For this review, take the finished solid that the model builds, in its own axes (mm). Face numbers are marked on the shaded views. A direction names the side the tool comes from. Coordinates: 2 decimals unless noted, no trailing zeros. Loops run counter-clockwise (first coordinate to the right, second up) from the corner with the lowest first, then second, coordinate; pieces in that order, holes last. Notation, with made-up numbers: (-16, 40.25) -> (39, 40.25) arc R21 ccw to (39, 77.25) -> close; hole circle Ø5 at (50.25, -38.75). An arc over 180 degrees is marked (long way). Answer in a Markdown table with one row per item.
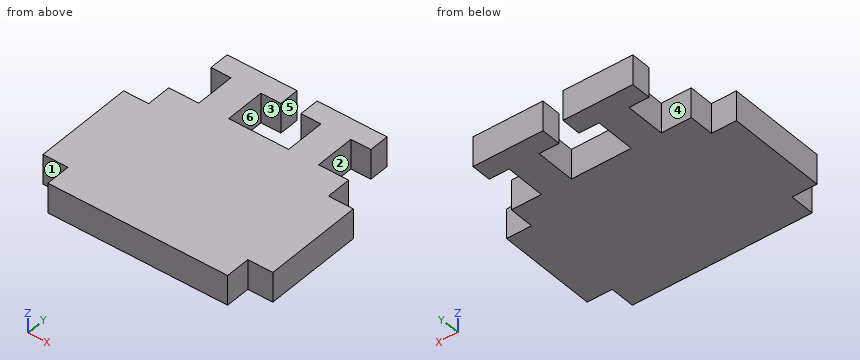
Autodesk Inventor part; units mm, degrees
ref_plane "YZ Plane" through (0, 0, 0) normal (1, 0, 0) x (0, 1, 0)
ref_plane "XZ Plane" through (0, 0, 0) normal (0, 1, 0) x (-1, 0, 0)
ref_plane "XY Plane" through (0, 0, 0) normal (0, 0, 1) x (1, 0, 0)
sketch "Sketch1" plane through (0, 0, 0) normal (0, 0, 1) x (1, 0, 0)
  line L0 (0, 0) -> (18, 0)
  line L1 (18, 0) -> (18, 15)
  line L2 (18, 15) -> (0, 15)
  line L3 (0, 15) -> (0, 0)
  line L4 (20.5, 12.5) -> (18, 12.5)
  line L5 (18, 12.5) -> (18, 2.5)
  line L6 (18, 2.5) -> (20.5, 2.5)
  line L7 (20.5, 2.5) -> (20.5, 12.5)
  line L8 (20.5, 12.5) -> (18, 2.5) construction
  line L9 (18, 12.5) -> (20.5, 2.5) construction
  line L10 (-2.5, 12.5) -> (0, 12.5)
  line L11 (0, 12.5) -> (0, 2.5)
  line L12 (0, 2.5) -> (-2.5, 2.5)
  line L13 (-2.5, 2.5) -> (-2.5, 12.5)
  line L14 (-2.5, 12.5) -> (0, 2.5) construction
  line L15 (0, 12.5) -> (-2.5, 2.5) construction
  line L16 (3, 15) -> (3, 19)
  line L17 (3, 19) -> (1, 19)
  line L18 (1, 19) -> (1, 21)
  line L19 (1, 21) -> (8, 21)
  line L20 (8, 21) -> (8, 19)
  line L21 (8, 19) -> (6, 19)
  line L22 (6, 19) -> (6, 15)
  line L23 (12, 15) -> (12, 19)
  line L24 (12, 19) -> (10, 19)
  line L25 (10, 19) -> (10, 21)
  line L26 (10, 21) -> (17, 21)
  line L27 (17, 21) -> (17, 19)
  line L28 (17, 19) -> (15, 19)
  line L29 (15, 19) -> (19.0944, 19)
  line L30 (15, 19) -> (15, 15)
  point P0 (19.25, 7.5)
  point P1 (-1.25, 7.5)
  point P2 (18, 7.5)
  point P3 (0, 7.5)
  point P4 (0, 12.5)
  dimension "d0" = 18
  dimension "d1" = 15
  dimension "d2" = 2.5
  dimension "d3" = 2.5
  dimension "d4" = 10
  dimension "d5" = 4
  dimension "d6" = 2
  dimension "d7" = 2
  dimension "d8" = 7
  dimension "d9" = 2
  dimension "d10" = 2
  dimension "d11" = 3
  dimension "d21" = 4
  dimension "d22" = 2
  dimension "d23" = 2
  dimension "d24" = 7
  dimension "d25" = 2
  dimension "d26" = 2
  dimension "d27" = 3
extrude "Extrusion1" add sketch "Sketch1" along normal blind 3
properties part number "Spring_holder2"
Item 1: Take a section at A-A, the plane y = 17.75. State the section outline as (x, z) points.
Worked answers:
| item | result |
|---|---|
| outline | (3, 0) -> (6, 0) -> (6, 3) -> (3, 3) -> close; (12, 0) -> (15, 0) -> (15, 3) -> (12, 3) -> close |
Item 2: The part is to be moulded in two halves that separate along X. For the marked faces 1, 2 and 3, say which applies: +X half, -X half, draft (parallel to the pull), parting line (faces both ways), or undercut.
Worked answers:
| item | result |
|---|---|
| face 1 | draft |
| face 2 | +X half |
| face 3 | undercut |
Item 3: Take a section at B-B, the plane x = 7.25. State the section outline as (y, z) points.
Worked answers:
| item | result |
|---|---|
| outline | (0, 0) -> (15, 0) -> (15, 3) -> (0, 3) -> close; (19, 0) -> (21, 0) -> (21, 3) -> (19, 3) -> close |
Item 4: Take a section at D-D, the plane y = 13.25. State the section outline as (x, z) points, and give its area (3 significant figures).
Worked answers:
| item | result |
|---|---|
| outline | (0, 0) -> (18, 0) -> (18, 3) -> (0, 3) -> close |
| area | 54.0 mm² |
Item 5: Insertion check: pin 1 (1.5 mm diameter, centred on y = 16.5, z = 1, fed in from -X); pin 2 (1.5 mm diameter, centred on y = 18, z = 1, fed in from +X); pin 3 (1 mm diameter, centred on y = 20, z = 1.5, fed in from -X); pin 4 (1 mm diameter, centred on x = 11, z = 1.5, fed in from -Y). Each pin has a flat end and moves straight along its axis. Give the tip position at first contact, or say it passes through.
Worked answers:
| item | result |
|---|---|
| pin 1 | x = 3 |
| pin 2 | x = 15 |
| pin 3 | x = 1 |
| pin 4 | y = 0 |
Item 6: For the marked faces 4, 5 and 6, list the 3-axis set-ups (+Z, -Z, +X, -X, +Y, -Y) from which the entire face can be reached by the end or side of a thin tool; tool diameter is ignored.
Worked answers:
| item | result |
|---|---|
| face 4 | +Z, -Z, -X |
| face 5 | +Z, -Z, +Y |
| face 6 | +Z, -Z |
Item 7: Take a section at C-C, the plane z = 1.55. State the section outline as (x, y) points.
Worked answers:
| item | result |
|---|---|
| outline | (-2.5, 2.5) -> (0, 2.5) -> (0, 0) -> (18, 0) -> (18, 2.5) -> (20.5, 2.5) -> (20.5, 12.5) -> (18, 12.5) -> (18, 15) -> (15, 15) -> (15, 19) -> (17, 19) -> (17, 21) -> (10, 21) -> (10, 19) -> (12, 19) -> (12, 15) -> (6, 15) -> (6, 19) -> (8, 19) -> (8, 21) -> (1, 21) -> (1, 19) -> (3, 19) -> (3, 15) -> (0, 15) -> (0, 12.5) -> (-2.5, 12.5) -> close |
Item 8: For L1, parallel to X at y = 17, z = 2.7; L2, parallel to X at y = 19.25, z = 0.25; L3, parallel to Y at x = 2.75, z = 2.1, list the stretches that pass through material, from the lowest coordinate up.
Worked answers:
| item | result |
|---|---|
| L1 | 3 to 6, 12 to 15 |
| L2 | 1 to 8, 10 to 17 |
| L3 | 0 to 15, 19 to 21 |
